Design review of the part built by this model. Coordinates are the model's own, in mm. A direction names the side the tool comes from. Coordinates: 2 decimals unless noted, no trailing zeros. Loops run counter-clockwise (first coordinate to the right, second up) from the corner with the lowest first, then second, coordinate; pieces in that order, holes last.
Q1. Machinability: for faces 4 (the face through (26.317, -8.287, 2.667)), 5 (the face through (26.5, -8.34, 58.47)), 6 (the face through (15, 14, -49.918)), which of the approach directions +Z, -Z, +X, -X, +Y, -Y give a long, thin tool a straight path to every point of the face, cutting with its end or side? Answer none if there is none.
Q2. Add section C-C on z = 28. Give the boundary of the cut face in (x, y), and give its area (3 significant figures).
Q3. Wall thickness on probe 1 along Y at (x, z) = (-1, -32.5); probe 2 along Y at (x, z) = (0, 50); probe 3 along Z at (x, y) = (-24.5, 4): over which ranges is each line inside the solid? List them lowest first.
Q4. Add section A-A on x = 0. Give the boundary of the cut face in (y, z), and give its area (3 significant figures).
Q5. Draft analysis for pull direction X (two halves, no side actions). For faces 1 (the face through (2, 25, 55.65)), 2 (the face through (23.47, -7.39, 50.17)), 3 (the face through (18.927, -5.961, 49.134)), state which applies: released by +X, released by -X, zero draft, split by the parting line, or undercut.
Q6. For P1, Ø2, axis at y = 21, z = 32.5, coming from the -X side; P2, Ø19, axis at x = -14.5, y = 0, coming from the +Z side; P3, Ø10, axis at x = 2.5, z = 7, coming from the -Y side; P4, Ø6, axis at y = -23.5, z = 2.5, coming from the +X side, all flat-tipped, find the tip position at first contact; note any pin that passes through.
```python
from build123d import *

# Parameters (mm, degrees)
FILLET1_R = 0.79375


with BuildPart() as part:
    # Sketch1 → Revolve1 (revolve)
    with BuildSketch(Plane(origin=(0, 0, 0), x_dir=(0, 0, -1), z_dir=(1, 0, 0)), mode=Mode.PRIVATE) as revolve1_sk:
        Polygon((-61.206526461, 19.84375), (-37.394026461, 19.84375), (-37.394026461, 18.794647739), (49.918473539, 18.794647739), (49.918473539, 31.75), (40.393473539, 31.75), (40.393473539, 27.590649684), (-44.537776461, 27.590649684), (-44.537776461, 24.60625), (-55.650276461, 24.60625), (-55.650276461, 27.78125), (-61.206526461, 27.78125), align=None)
    revolve(revolve1_sk.sketch.rotate(Axis((0, 0, 20.539691943), (0, 0, -1)), 90), axis=Axis((0, 0, 20.539691943), (0, 0, -1)))

    # Fillet1
    fillet1_edges = [part.edges().sort_by_distance(p)[0] for p in [
        (-18.794647739, 0, -49.918473539),
    ]]
    fillet(fillet1_edges, radius=FILLET1_R)


solid = part.part
```
Entries:
1. face 4: none
1. face 5: +Z
1. face 6: -Z, +X, -X, +Y, -Y
2. outline: circle Ø55.18 at (0, 0); hole circle Ø37.59 at (0, 0)
2. area: 1,280 mm2
3. probe 1: y = -27.57 to -18.77, 18.77 to 27.57
3. probe 2: y = -24.61 to -19.84, 19.84 to 24.61
3. probe 3: z = -49.92 to 44.54, 55.65 to 61.21
4. outline: (-31.75, -49.92) - (-19.59, -49.92) arc R0.79 ccw to (-18.79, -49.12) - (-18.79, 37.39) - (-19.84, 37.39) - (-19.84, 61.21) - (-27.78, 61.21) - (-27.78, 55.65) - (-24.61, 55.65) - (-24.61, 44.54) - (-27.59, 44.54) - (-27.59, -40.39) - (-31.75, -40.39) - close; (18.79, -49.12) arc R0.79 ccw to (19.59, -49.92) - (31.75, -49.92) - (31.75, -40.39) - (27.59, -40.39) - (27.59, 44.54) - (24.61, 44.54) - (24.61, 55.65) - (27.78, 55.65) - (27.78, 61.21) - (19.84, 61.21) - (19.84, 37.39) - (18.79, 37.39) - close
4. area: 1,920 mm2
5. face 1: zero draft
5. face 2: split by the parting line
5. face 3: undercut
6. P1: stops at x = -19.01
6. P2: stops at z = 61.21
6. P3: stops at y = -27.59
6. P4: stops at x = 18.47
